```python
from build123d import *

# Parameters (mm, degrees)
BOSS_EXTRUDE1_DEPTH = 9.4
BOSS_EXTRUDE2_DEPTH = 20
BOSS_EXTRUDE4_DEPTH = 8.6
SKETCH5_R           = 11
BOSS_EXTRUDE5_DEPTH = 2
SKETCH6_R           = 2.5
CUT_EXTRUDE1_DEPTH  = 2
BOSS_EXTRUDE6_DEPTH = 23.5
SKETCH8_W           = 16.2
SKETCH8_H           = 1.444611315
BOSS_EXTRUDE7_DEPTH = 5.08
SKETCH9_R           = 1.5
CUT_EXTRUDE2_DEPTH  = 4.5


with BuildPart() as part:
    # Sketch1 → Boss-Extrude1 (new body)
    with BuildSketch(Plane.XY):
        with BuildLine():
            Line((-16.07, -21.15), (16.07, -21.15))
            ThreePointArc((16.07, -21.15), (19.662102448, -19.662102448), (21.15, -16.07))
            Line((21.15, -16.07), (21.15, 16.07))
            ThreePointArc((21.15, 16.07), (19.662102448, 19.662102448), (16.07, 21.15))
            Line((16.07, 21.15), (-16.07, 21.15))
            ThreePointArc((-16.07, 21.15), (-19.662102448, 19.662102448), (-21.15, 16.07))
            Line((-21.15, 16.07), (-21.15, -16.07))
            ThreePointArc((-21.15, -16.07), (-19.662102448, -19.662102448), (-16.07, -21.15))
        make_face()
    extrude(amount=BOSS_EXTRUDE1_DEPTH)

    # Sketch2 → Boss-Extrude2 (add)
    with BuildSketch(Plane.XY.offset(9.4)):
        with BuildLine():
            Line((-14.582102448, -19.662102448), (14.582102448, -19.662102448))
            ThreePointArc((14.582102448, -19.662102448), (18.174204897, -18.174204897), (19.662102448, -14.582102448))
            Line((19.662102448, -14.582102448), (19.662102448, 14.582102448))
            ThreePointArc((19.662102448, 14.582102448), (18.174204897, 18.174204897), (14.582102448, 19.662102448))
            Line((14.582102448, 19.662102448), (-14.582102448, 19.662102448))
            ThreePointArc((-14.582102448, 19.662102448), (-18.174204897, 18.174204897), (-19.662102448, 14.582102448))
            Line((-19.662102448, 14.582102448), (-19.662102448, -14.582102448))
            ThreePointArc((-19.662102448, -14.582102448), (-18.174204897, -18.174204897), (-14.582102448, -19.662102448))
        make_face()
    extrude(amount=BOSS_EXTRUDE2_DEPTH)

    # Sketch4 → Boss-Extrude4 (add)
    with BuildSketch(Plane.XY.offset(29.4)):
        with BuildLine():
            Line((16.129, -21.209), (-16.129, -21.209))
            ThreePointArc((-16.129, -21.209), (-19.721102448, -19.721102448), (-21.209, -16.129))
            Line((-21.209, -16.129), (-21.209, 16.129))
            ThreePointArc((-21.209, 16.129), (-19.721102448, 19.721102448), (-16.129, 21.209))
            Line((-16.129, 21.209), (16.129, 21.209))
            ThreePointArc((16.129, 21.209), (19.721102448, 19.721102448), (21.209, 16.129))
            Line((21.209, 16.129), (21.209, -16.129))
            ThreePointArc((21.209, -16.129), (19.721102448, -19.721102448), (16.129, -21.209))
        make_face()
    extrude(amount=BOSS_EXTRUDE4_DEPTH)

    # Sketch5 → Boss-Extrude5 (add)
    with BuildSketch(Plane.XY.offset(38)):
        Circle(SKETCH5_R)
    extrude(amount=BOSS_EXTRUDE5_DEPTH)

    # Sketch6 → Cut-Extrude1 (cut)
    with BuildSketch(Plane.XY.offset(40)):
        Circle(SKETCH6_R)
    extrude(amount=-CUT_EXTRUDE1_DEPTH, mode=Mode.SUBTRACT)

    # Sketch7 → Boss-Extrude6 (add)
    with BuildSketch(Plane.XY.offset(38)):
        with BuildLine():
            Line((1.876071115, 1.242118018), (-1.876071115, 1.242118018))
            ThreePointArc((-1.876071115, 1.242118018), (0, -2.25), (1.876071115, 1.242118018))
        make_face()
    extrude(amount=BOSS_EXTRUDE6_DEPTH)

    # Sketch8 → Boss-Extrude7 (add)
    with BuildSketch(Plane(origin=(0, 21.15, 0), x_dir=(1, 0, 0), z_dir=(0, 1, 0))):
        with Locations((0, -1.343147685)):
            Rectangle(SKETCH8_W, SKETCH8_H)
    extrude(amount=BOSS_EXTRUDE7_DEPTH)

    # Sketch9 → Cut-Extrude2 (cut)
    with BuildSketch(Plane.XY.offset(38)):
        with Locations((-15.559, 15.559)):
            Circle(SKETCH9_R)
        with Locations((15.559, 15.559)):
            Circle(SKETCH9_R)
        with Locations((15.559, -15.559)):
            Circle(SKETCH9_R)
        with Locations((-15.559, -15.559)):
            Circle(SKETCH9_R)
    extrude(amount=-CUT_EXTRUDE2_DEPTH, mode=Mode.SUBTRACT)


solid = part.part
```
Input: part model. Units: mm. Frame: model coordinates. A direction names the side the tool comes from. Give positions to 0.01 mm unless a question says otherwise; leave off trailing zeros. Loops run counter-clockwise (first coordinate to the right, second up) from the corner with the lowest first, then second, coordinate; pieces in that order, holes last. Notation, with made-up numbers: M 39,8.5 L 82,8.5 A17 ccw 82,30.5 Z; hole C -8.5,-15 d8. An arc over 180 degrees is marked long. Answer as CSV lines item,"result". Start each with the question number.
1. Section D-D on x = 0. Return loops of the section in (y, z), plus the area to 3 significant figures.
2. Section A-A on z = 12.5. Return loops of the section in (x, y).
3. Reachability of faces 5 (the face through (-17.058, -15.493, 35.782)), 6 (the face through (18.134, -18.213, 19.26)), 7 (the face through (0, -21.15, 5)), 8 (the face through (-19.662, 0, 19)) from +Z, -Z, +X, -X, +Y, -Y: full face, straight path, thin tool, end or side. Return the list, or none.
4. Pull-direction query (Y, two-part tool) for faces 1 (the face through (-15.9, 14.1, 35.8)), 2 (the face through (0, 19.662, 19)), 3 (the face through (16, 16, 33.5)), 4 (the face through (21.15, 0, 5)); classes: released by +Y, released by -Y, zero draft, split by the parting line, or undercut.
5. Section B-B on x = -12. Return loops of the section in (y, z).
6. Pin query (flat end, axial travel): P1, Ø3, axis at x = 8, z = 22.5, coming from the +Y side; P2, Ø4, axis at x = -2.5, y = 22.5, coming from the +Z side; P3, Ø1.5, axis at x = 13.5, z = 10, coming from the +Y side. Return the tip coordinate at first contact, or that it passes through.
7. Line query: L1, parallel to Y at x = 0, z = 39; L2, parallel to Y at x = 8, z = 19.5; L3, parallel to Y at x = 15, z = 27.5. Output: solid intervals per line, ascending.
8. Section C-C on y = 0. Return loops of the section in (x, z).
Computed values:
1,outline,"M -21.21,29.4 L -19.66,29.4 L -19.66,9.4 L -21.15,9.4 L -21.15,0 L 21.15,0 L 21.15,0.62 L 26.23,0.62 L 26.23,2.07 L 21.15,2.07 L 21.15,9.4 L 19.66,9.4 L 19.66,29.4 L 21.21,29.4 L 21.21,38 L 11,38 L 11,40 L 2.5,40 L 2.5,38 L 1.24,38 L 1.24,61.5 L -2.25,61.5 L -2.25,38 L -2.5,38 L -2.5,40 L -11,40 L -11,38 L -21.21,38 Z"
1,area,"1,670 mm²"
2,outline,"M -19.66,-14.58 A5.08 ccw -14.58,-19.66 L 14.58,-19.66 A5.08 ccw 19.66,-14.58 L 19.66,14.58 A5.08 ccw 14.58,19.66 L -14.58,19.66 A5.08 ccw -19.66,14.58 Z"
3,face 5,"+Z"
3,face 6,"+X, -Y"
3,face 7,"-Z, +X, -X, -Y"
3,face 8,"-X, +Y, -Y"
4,face 1,"undercut"
4,face 2,"released by +Y"
4,face 3,"undercut"
4,face 4,"zero draft"
5,outline,"M -21.21,29.4 L -19.66,29.4 L -19.66,9.4 L -21.15,9.4 L -21.15,0 L 21.15,0 L 21.15,9.4 L 19.66,9.4 L 19.66,29.4 L 21.21,29.4 L 21.21,38 L -21.21,38 Z"
6,P1,"stops at y = 19.66"
6,P2,"stops at z = 38"
6,P3,"stops at y = 21.15"
7,L1,"y = -11 to -2.5, -2.25 to 1.24, 2.5 to 11"
7,L2,"y = -19.66 to 19.66"
7,L3,"y = -19.64 to 19.64"
8,outline,"M -21.21,29.4 L -19.66,29.4 L -19.66,9.4 L -21.15,9.4 L -21.15,0 L 21.15,0 L 21.15,9.4 L 19.66,9.4 L 19.66,29.4 L 21.21,29.4 L 21.21,38 L 11,38 L 11,40 L 2.5,40 L 2.5,38 L 2.25,38 L 2.25,61.5 L -2.25,61.5 L -2.25,38 L -2.5,38 L -2.5,40 L -11,40 L -11,38 L -21.21,38 Z"
